Could you check a few things on this model? Use its own coordinates, in mm. A direction names the side the tool comes from. Coordinates: 2 decimals unless noted, no trailing zeros. Write each loop counter-clockwise with the first axis right and the second up, starting at its lowest first coordinate (ties: lowest second). Pieces come first, ordered by that corner, then holes.
Item 1: Thinking about a two-plate mould opening in Y: for faces 1 (the flat face through (-3.3, 0, 3)), 2 (the cylindrical face through (-0.026, -6.529, 12.553)), 3 (the cylindrical face through (0.046, 10.342, -4.914)), which applies, +Y half, -Y half, draft (parallel to the pull), parting line (faces both ways), or undercut?
Item 2: If I drill on probe 1 along Y at (x, z) = (0, -5.75); probe 2 along Y at (x, z) = (-0.25, 0.25); probe 3 along Y at (x, z) = (-2, 0.5), over which ranges is the centre line in solid material (lowest first)?
Item 3: Which directions (+Z, -Z, +X, -X, +Y, -Y) give clear straight access to the entire face, cutting with the end or side of a thin tool? Please do faces 4 (the cylindrical face through (1.06, -0.18, -1.49)), 5 (the cylindrical face through (-2.59, 1.7, -12.94)), 6 (the cylindrical face through (2.56, 1.7, -12.94)).
Item 4: For P1, Ø1, axis at x = 3, y = -3.5, coming from the +Z side; P2, Ø5, axis at x = 0.5, z = 11, coming from the -Y side, each with a flat end and sliding along its axis, tell me the tip position at first contact or that it passes through.
Item 5: I want a section at A-A on y = -6.25. Please give me the cut outline in (x, z).
Item 6: I want a section at D-D on x = 4.5. Please give me the cut outline in (y, z).
Item 7: I want a section at C-C on y = -9.5. Please give me the cut outline in (x, z).
Item 8: I want a section at B-B on x = 2.5. State how many separate pieces and enclosed holes the cut face has, then the cut area to 3 significant figures.
from build123d import *

# Parameters (mm, degrees)
ODEBRAT_VYSUNUT_M1_DEPTH = 10
ZAOBLIT1_R               = 1
ZAOBLIT2_R               = 1
ZAOBLIT4_R               = 1
ODEBRAT_VYSUNUT_M2_DEPTH = 10
P_IDAT_START             = 2
P_IDAT_VYSUNUT_M1_DEPTH  = 2
ZAOBLIT5_R               = 0.2


with BuildPart() as part:
    # Skica1 → Rotovat1 (revolve)
    with BuildSketch(Plane.XY, mode=Mode.PRIVATE) as rotovat1_sk:
        Polygon((1.849988347, 14.15), (-1.849988347, 14.15), (-1.849988347, 13.05), (-3.3, 13.05), (-3.3, 0), (3.3, 0), (3.3, 13.05), (1.849988347, 13.05), align=None)
    revolve(rotovat1_sk.sketch.rotate(Axis((-3.3, 0, 0), (1, 0, 0)), 180), axis=Axis((-3.3, 0, 0), (1, 0, 0)))

    # Skica2 → Odebrat vysunutím1 (cut)
    with BuildSketch(Plane(origin=(3.3, 0, 0), x_dir=(0, 0, -1), z_dir=(1, 0, 0))):
        with BuildLine():
            ThreePointArc((-1.725, 2.987787643), (1.446819914, 3.131966177), (3.393206272, 0.623418956))
            Line((3.393206272, 0.623418956), (11.018835658, 3.112516786))
            ThreePointArc((11.018835658, 3.112516786), (4.801764642, 10.394496444), (-4.773151875, 10.407666462))
            Line((-4.773151875, 10.407666462), (-1.725, 2.987787643))
        make_face()
        with BuildLine():
            ThreePointArc((-1.725, -2.987787643), (-3.43577223, -0.313000288), (-2.236499789, 2.626893354))
            Line((-2.236499789, 2.626893354), (-8.204936435, 7.986333207))
            ThreePointArc((-8.204936435, 7.986333207), (-11.402780301, -1.038798059), (-6.626727613, -9.33750401))
            Line((-6.626727613, -9.33750401), (-1.725, -2.987787643))
        make_face()
        with BuildLine():
            Line((11.399879487, -1.070162452), (3.45, 0))
            ThreePointArc((3.45, 0), (1.988952316, -2.818965889), (-1.156706483, -3.25031231))
            Line((-1.156706483, -3.25031231), (-2.813899223, -11.098849993))
            ThreePointArc((-2.813899223, -11.098849993), (6.601015659, -9.355698385), (11.399879487, -1.070162452))
        make_face()
    extrude(amount=-ODEBRAT_VYSUNUT_M1_DEPTH, mode=Mode.SUBTRACT)

    # Zaoblit1
    zaoblit1_edges = [part.edges().sort_by_distance(p)[0] for p in [
        (0, 7.986333207, 8.204936435),
    ]]
    fillet(zaoblit1_edges, radius=ZAOBLIT1_R)

    # Zaoblit2
    zaoblit2_edges = [part.edges().sort_by_distance(p)[0] for p in [
        (0, 10.407666462, 4.773151875),
        (0, 3.112516786, -11.018835658),
        (0, -9.33750401, 6.626727613),
        (0, -1.070162452, -11.399879487),
        (0, -11.098849993, 2.813899223),
    ]]
    fillet(zaoblit2_edges, radius=ZAOBLIT2_R)

    # Zaoblit4
    zaoblit4_edges = [part.edges().sort_by_distance(p)[0] for p in [
        (0, 0.623418956, -3.393206272),
        (0, 2.987787643, 1.725),
        (0, 2.626893354, 2.236499789),
        (0, -2.987787643, 1.725),
        (0, -3.25031231, 1.156706483),
        (0, 0, -3.45),
    ]]
    fillet(zaoblit4_edges, radius=ZAOBLIT4_R)

    # Skica3 → Odebrat vysunutím2 (cut)
    with BuildSketch(Plane(origin=(3.3, 0, 0), x_dir=(0, 0, -1), z_dir=(1, 0, 0))):
        with BuildLine():
            Line((1.046984184, 1.074162054), (1.885452924, 2.889215684))
            ThreePointArc((1.885452924, 2.889215684), (1.446819914, 3.131966177), (0.977636641, 3.308583775))
            Line((0.977636641, 3.308583775), (0.1391679, 1.493530146))
            ThreePointArc((0.1391679, 1.493530146), (-1.149085352, 0.964159143), (-1.446658447, -0.396458495))
            Line((-1.446658447, -0.396458495), (0.78566452, -1.277783731))
            ThreePointArc((0.78566452, -1.277783731), (1.490826134, -0.165642502), (1.046984184, 1.074162054))
        make_face()
    extrude(amount=-ODEBRAT_VYSUNUT_M2_DEPTH, mode=Mode.SUBTRACT)

    # Skica5 → Přidat vysunutím1 (add)
    with BuildSketch(Plane(origin=(3.3, 0, 0), x_dir=(0, 0, -1), z_dir=(1, 0, 0)).offset(P_IDAT_START)):
        with BuildLine():
            Line((0.977636641, 3.308583775), (0.1391679, 1.493530146))
            ThreePointArc((0.1391679, 1.493530146), (-1.149085352, 0.964159143), (-1.446658447, -0.396458495))
            Line((-1.446658447, -0.396458495), (0.78566452, -1.277783731))
            ThreePointArc((0.78566452, -1.277783731), (1.490826134, -0.165642502), (1.046984184, 1.074162054))
            Line((1.046984184, 1.074162054), (1.885452924, 2.889215684))
            ThreePointArc((1.885452924, 2.889215684), (-1.446819914, -3.131966177), (0.977636641, 3.308583775))
        make_face()
    extrude(amount=-P_IDAT_VYSUNUT_M1_DEPTH)

    # Zaoblit5
    zaoblit5_edges = [part.edges().sort_by_distance(p)[0] for p in [
        (5.3, -3.131966177, 1.446819914),
    ]]
    fillet(zaoblit5_edges, radius=ZAOBLIT5_R)


solid = part.part
Response values:
1. face 1: draft
1. face 2: parting line
1. face 3: undercut
2. probe 1: y = -12.93 to -9.9, -0.31 to 1.39, 9.9 to 12.93
2. probe 2: y = -14.15 to -11.45, -3.44 to -0.87, 1.48 to 3.44, 11.45 to 14.15
2. probe 3: y = -13.04 to -11.44, -3.44 to -0.77, 1.41 to 3.41, 11.44 to 13.04
3. face 4: +X, -X
3. face 5: -X
3. face 6: +X
4. P1: stops at z = 12.7
4. P2: stops at y = -11.31
5. outline: (-3.3, -11.46) - (-1.85, -11.46) - (-1.85, -12.69) - (1.85, -12.69) - (1.85, -11.46) - (3.3, -11.46) - (3.3, -9.59) - (-3.3, -9.59) - close; (-3.3, 1.79) - (3.3, 1.79) - (3.3, 4.24) - (-3.3, 4.24) - close; (-3.3, 9.59) - (3.3, 9.59) - (3.3, 11.46) - (1.85, 11.46) - (1.85, 12.69) - (-1.85, 12.69) - (-1.85, 11.46) - (-3.3, 11.46) - close
6. outline: (-1.28, -0.79) - (-0.4, 1.45) arc R1.5 cw to (1.49, -0.14) - (3.31, -0.98) arc R3.45 ccw (long way) to (2.89, -1.89) - (1.07, -1.05) arc R1.5 cw to start
7. outline: (-3.3, -8.95) - (-1.85, -8.95) - (-1.85, -10.49) - (1.85, -10.49) - (1.85, -8.95) - (3.3, -8.95) - (3.3, -6.39) - (-3.3, -6.39) - close; (-3.3, 2.48) - (3.3, 2.48) - (3.3, 8.95) - (1.85, 8.95) - (1.85, 10.49) - (-1.85, 10.49) - (-1.85, 8.95) - (-3.3, 8.95) - close
8. separate pieces: 1
8. enclosed holes: 3
8. area: 213 mm2
